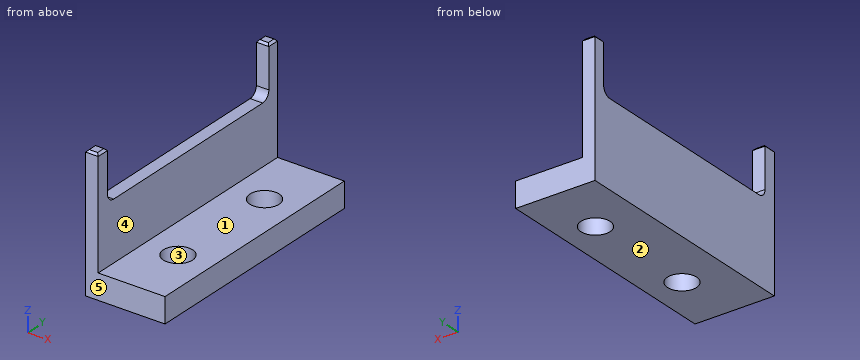
from build123d import *

# Parameters (mm, degrees)
F1_DEPTH = 3
F2_W     = 1.5
F2_H     = 29
F3_DEPTH = 13
F5_D     = 3.5
F7_DEPTH = 1.501
F8_R     = 1
F9_SIZE  = 0.25


with BuildPart() as f1:
    # F0 (on Top) → F1 (new body)
    with BuildSketch(Plane.XY):
        Polygon((0, 29), (0, 0), (9.5, 0), (9.5, 29), (1.5, 29), align=None)
    extrude(amount=F1_DEPTH)

    # F2 (on face) → F3 (join)
    with BuildSketch(Plane.XY.offset(3)):
        with Locations((0.75, 14.5)):
            Rectangle(F2_W, F2_H)
    extrude(amount=F3_DEPTH)

    # F5 (through all)
    with Locations(Plane.XY.offset(3)):
        with Locations((5.5, 21.5), (5.5, 7.5)):
            Hole(F5_D / 2)

    # F6 (on face) → F7 (cut, through all)
    with BuildSketch(Plane.YZ.offset(1.5)):
        Polygon((27.5, 16), (1.5, 16), (1.5, 10), (27.5994203985, 10), (27.5994203985, 16), align=None)
    extrude(amount=-F7_DEPTH, mode=Mode.SUBTRACT)

    # F8
    f8_edges = [f1.edges().sort_by_distance(p)[0] for p in [
        (0.75, 27.59942, 10),
        (0.75, 1.5, 10),
    ]]
    fillet(f8_edges, radius=F8_R)

    # F9
    f9_edges = [f1.edges().sort_by_distance(p)[0] for p in [
        (0.75, 27.59942, 16),
        (1.5, 28.29971, 16),
        (0.75, 29, 16),
        (0, 28.29971, 16),
        (0.75, 1.5, 16),
        (1.5, 0.75, 16),
        (0.75, 0, 16),
        (0, 0.75, 16),
    ]]
    chamfer(f9_edges, length=F9_SIZE)


solid = f1.part
Could you check a few things on this model? Use its own coordinates, in mm. Face numbers are marked on the shaded views. A direction names the side the tool comes from. Round coordinates to 2 decimals unless told otherwise and drop trailing zeros. Order: outer loops, then holes, each group sorted by start corner. A loop starts at its lowest first (then second) coordinate and runs counter-clockwise, first axis right, second up.
Q1. Which directions (+Z, -Z, +X, -X, +Y, -Y) give clear straight access to the entire face, cutting with the end or side of a thin tool? Please do the marked faces 1 and 2.
Geometry says:
face 1: +Z, +X, +Y, -Y
face 2: -Z, +X, -X, +Y, -Y
Q2. I'm going to push flat-ended pins straight in: P1, Ø1.2, axis at x = 0.5, y = 9, coming from the +Z side; P2, Ø2, axis at x = 6, y = 18, coming from the +Z side; P3, Ø3, axis at y = 19.5, z = 6, coming from the +X side. Where does each tip first touch, or does it pass through?
Geometry says:
P1: stops at z = 10
P2: stops at z = 3
P3: stops at x = 1.5
Q3. Imagine slicing it at C-C, the plane y = 21.5. List the corners of the cut face in (x, z) for me.
Geometry says:
outline: (0, 0) - (3.75, 0) - (3.75, 3) - (1.5, 3) - (1.5, 10) - (0, 10) - close; (7.25, 0) - (9.5, 0) - (9.5, 3) - (7.25, 3) - close
Q4. Thinking about a two-plate mould opening in Y: for the marked faces 3, 4 and 5, which applies, released by +Y, released by -Y, zero draft, split by the parting line, or undercut?
Geometry says:
face 3: undercut
face 4: zero draft
face 5: released by -Y
Q5. Imagine slicing it at B-B, the plane z = 13.25. List the corners of the cut face in (x, y) for me.
Geometry says:
outline: (0, 0) - (1.5, 0) - (1.5, 1.5) - (0, 1.5) - close; (0, 27.6) - (1.5, 27.6) - (1.5, 29) - (0, 29) - close
Q6. Imagine slicing it at D-D, the plane y = 4.5. List the corners of the cut face in (x, z) for me, then the cut area to 3 significant figures.
Geometry says:
outline: (0, 0) - (9.5, 0) - (9.5, 3) - (1.5, 3) - (1.5, 10) - (0, 10) - close
area: 39.0 mm2
Q7. Imagine slicing it at A-A, the plane x = 5.5. List the corners of the cut face in (y, z) for me.
Geometry says:
outline: (0, 0) - (5.75, 0) - (5.75, 3) - (0, 3) - close; (9.25, 0) - (19.75, 0) - (19.75, 3) - (9.25, 3) - close; (23.25, 0) - (29, 0) - (29, 3) - (23.25, 3) - close
Q8. Please list where these lines run through material, in increasing order: probe 1 along Y at (x, z) = (5.5, 0.75); probe 2 along Z at (x, y) = (3.5, 12.5); probe 3 along Y at (x, z) = (4, 1.25).
Geometry says:
probe 1: y = 0 to 5.75, 9.25 to 19.75, 23.25 to 29
probe 2: z = 0 to 3
probe 3: y = 0 to 6.6, 8.4 to 20.6, 22.4 to 29
